Could you check a few things on this model? Use its own coordinates, in mm. A direction names the side the tool comes from. Give positions to 0.01 mm unless a question says otherwise; leave off trailing zeros. Write each loop counter-clockwise with the first axis right and the second up, starting at its lowest first coordinate (ties: lowest second). Pieces come first, ordered by that corner, then holes. Notation, with made-up numbers: M 43.5,44.5 L 68.5,44.5 A19 ccw 68.5,54.5 Z; hole C 24.25,-14 d7. An arc over 180 degrees is marked long. One line per item, written item: value.
Autodesk Inventor part; units mm, degrees
ref_plane "YZ Plane" through (0, 0, 0) normal (1, 0, 0) x (0, 1, 0)
ref_plane "XZ Plane" through (0, 0, 0) normal (0, 1, 0) x (-1, 0, 0)
ref_plane "XY Plane" through (0, 0, 0) normal (0, 0, 1) x (1, 0, 0)
sketch "Эскиз1" plane through (0, 0, 0) normal (0, 1, 0) x (-1, 0, 0)
  line L0 (-20, -17.5) -> (20, -17.5)
  line L1 (20, -17.5) -> (20, 17.5)
  line L2 (20, 17.5) -> (-20, 17.5)
  line L3 (-20, 17.5) -> (-20, -17.5)
  line L4 (-20, -17.5) -> (20, 17.5) construction
  line L5 (20, -17.5) -> (-20, 17.5) construction
  line L6 (-10, 17.5) -> (-10, -17.5) construction
  circle A0 centre (-10, 10) radius 1.5
  circle A1 centre (-10, -10) radius 1.5
  line L7 (0, 0) -> (-17.0059, 0) construction
  line L8 (5.5, -10.25) -> (16, -10.25)
  line L9 (16, -10.25) -> (16, 10.25)
  line L10 (16, 10.25) -> (5.5, 10.25)
  line L11 (5.5, 10.25) -> (5.5, -10.25)
  line L12 (5.5, -10.25) -> (16, 10.25) construction
  line L13 (16, -10.25) -> (5.5, 10.25) construction
  circle A2 centre (10.75, 0) radius 1.5
  point P0 (10.75, 0)
  point P1 (10.75, 0)
  dimension "d0" = 3
  dimension "d1" = 3
  dimension "d2" = 20
  dimension "d3" = 10
  dimension "d4" = 35
  dimension "d5" = 10.5
  dimension "d6" = 20.5
  dimension "d14" = 3
  dimension "d17" = 4
  dimension "d18" = 20
extrude "Выдавливание1" add sketch "Эскиз1" along normal blind 7 contours L3 L2 L1 L0
extrude "Выдавливание2" add sketch "Эскиз1" along normal blind 3.8 contours L11 L10 L9 L8 | A2
chamfer "Фаска1" distance 1.5 angle 45 2 edges at (11.5, 0, -10) (11.5, 0, 10)
extrude "Выдавливание3" add sketch "Эскиз1" along normal blind 6 contours A2
fillet "Сопряжение1" radius 5 1 edges at (20, 0, 0)
fillet "Сопряжение2" radius 5 1 edges at (-20, 0, 0)
sketch "Эскиз3" plane through (0, 0, 0) normal (0, -1, 0) x (1, 0, 0)
  line L0 (-15, 17.5) -> (15, 17.5)
  line L1 (-7, -17.5) -> (-13, -17.5)
  line L2 (-13, -17.5) -> (-13, 17.5)
  line L3 (-13, 17.5) -> (-7, 17.5)
  line L4 (-7, 17.5) -> (-7, -17.5)
  line L5 (-7, -17.5) -> (-13, 17.5) construction
  line L6 (-13, -17.5) -> (-7, 17.5) construction
  point P0 (0, 0)
  point P1 (-10, 0)
  dimension "d27" = 6
  dimension "d28" = 10
extrude "Выдавливание5" add sketch "Эскиз3" along normal blind 15
fillet "Сопряжение4" radius 10 2 edges at (-10, -15, 17.5) (-10, -15, -17.5)
fillet "Сопряжение5" radius 5 2 edges at (-13, 0, 0) (-7, 0, 0)
fillet "Сопряжение6" radius 2 22 edges at (-13, -15, 0) (-13, -12.0711, -14.5711) (-13, -4.7697, -17.5) (-13.9689, -1.5814, -17.5) (-19.0311, 2.042, -17.5) (-20, 6, -17.5) (-13, -4.7697, 17.5) (-13.9689, -1.5814, 17.5) (-19.0311, 2.042, 17.5) (-20, 6, 17.5) (-13, -12.0711, 14.5711) (-5.5355, -1.4645, 17.5) (6.5, 0, 17.5) (18.5355, 1.4645, 17.5) (20, 6, 17.5) (-7, -15, 0) (-7, -12.0711, -14.5711) (-5.5355, -1.4645, -17.5) (6.5, 0, -17.5) (18.5355, 1.4645, -17.5) (20, 6, -17.5) (-7, -12.0711, 14.5711)
sketch "Эскиз4" plane through (-10.75, 6, 0) normal (0, 1, 0) x (1, 0, 0)
  circle A0 centre (0, 0) radius 1.5
  point P0 (10.75, 0)
extrude "Выдавливание6" cut sketch "Эскиз4" against normal blind 10
properties part number "магнитный  держатель"
1) We'd pull the mould along X, two halves only. Please class faces 4 (the face through (19, 2, 0)), 5 (the face through (0, 4, -17.5)), 6 (the face through (10, 1, 12)): pulls with the +X half, pulls with the -X half, needs draft (parallel to the pull), parting line crosses it, or undercut.
Outcome:
face 4: pulls with the +X half
face 5: needs draft
face 6: undercut
2) On a 3-axis mill with a long thin cutter (end or side, diameter ignored), from which of +Z, -Z, +X, -X, +Y, -Y can I reach the whole of each face in a straight line? I mean faces 1 (the face through (7, 0, 0)), 2 (the face through (0, 4, 17.5)), 3 (the face through (-11, -4, 0)). Say none if no direction works.
Outcome:
face 1: +Z, -Z, +X, -Y
face 2: +Z, +X, -X, +Y, -Y
face 3: +Y
3) If we section it at A-A, the plane x = 10: Write out the boundary of the cut face in (y, z), then the cut area to 3 significant figures.
Outcome:
outline: M 0,-15.5 A2 ccw 2,-17.5 L 7,-17.5 L 7,-11.5 L 1.5,-11.5 L 0,-13 Z; M 0,-7 L 1.5,-8.5 L 7,-8.5 L 7,8.5 L 1.5,8.5 L 0,7 Z; M 0,13 L 1.5,11.5 L 7,11.5 L 7,17.5 L 2,17.5 A2 ccw 0,15.5 Z
area: 197 mm^2
4) Please list where these lines run through material, in increasing order: L1, parallel to Z at x = 10, y = 5.3; L2, parallel to Y at x = 4, z = -11; L3, parallel to Z at x = -10.75, y = -1.5. Write a range as from..to.
Outcome:
L1: z = -17.5..-11.5, -8.5..8.5, 11.5..17.5
L2: y = 0..7
L3: z = -17.5..-1.5, 1.5..17.5
5) If we section it at B-B, the plane x = 0.5: Write out the boundary of the cut face in (y, z), then the cut area to 3 significant figures.
Outcome:
outline: M 0,-15.5 A2 ccw 2,-17.5 L 7,-17.5 L 7,17.5 L 2,17.5 A2 ccw 0,15.5 Z
area: 243 mm^2
6) I'm going to push flat-ended pins straight in: pin 1 (7 mm diameter, centred on y = -7, z = 7, fed in from -X); pin 2 (5 mm diameter, centred on x = -10.75, z = 0, fed in from +Y); pin 3 (5 mm diameter, centred on y = -12, z = 8, fed in from +X). Where does each tip first touch, or does it pass through?
Outcome:
pin 1: stops at x = -13.11
pin 2: stops at y = 3.8
pin 3: stops at x = -7
